from build123d import *
from build123d.topology import SkipClean

# Parameters (mm, degrees)
BOSS_EXTRUDE1_DEPTH = 12
SKETCH2_R           = 0.5
BOSS_EXTRUDE2_DEPTH = 6
SKETCH3_W           = 80
SKETCH3_H           = 60
BOSS_EXTRUDE3_DEPTH = 5


with BuildPart() as part:
    # Sketch1 → Boss-Extrude1 (new body)
    with BuildSketch(Plane(origin=(19, 0, 0), x_dir=(0, 0, -1), z_dir=(1, 0, 0))):
        with BuildLine():
            Line((-17.5, 6.6), (-15.77498019, 6.6))
            ThreePointArc((-15.77498019, 6.6), (0, 17.1), (15.77498019, 6.6))
            Line((15.77498019, 6.6), (17.5, 6.6))
            ThreePointArc((17.5, 6.6), (24.1, 0), (17.5, -6.6))
            Line((17.5, -6.6), (15.77498019, -6.6))
            ThreePointArc((15.77498019, -6.6), (14.603463036, -8.896564918), (13.1, -10.990905331))
            Line((13.1, -10.990905331), (13.1, -12.489995997))
            ThreePointArc((13.1, -12.489995997), (11.807309956, -13.718506901), (10.4, -14.813844876))
            Line((10.4, -14.813844876), (10.4, -16))
            ThreePointArc((10.4, -16), (9.199137803, -18.899137803), (6.3, -20.1))
            Line((6.3, -20.1), (-6.3, -20.1))
            ThreePointArc((-6.3, -20.1), (-9.199137803, -18.899137803), (-10.4, -16))
            Line((-10.4, -16), (-10.4, -14.813844876))
            ThreePointArc((-10.4, -14.813844876), (-11.807309956, -13.718506901), (-13.1, -12.489995997))
            Line((-13.1, -12.489995997), (-13.1, -10.990905331))
            ThreePointArc((-13.1, -10.990905331), (-14.603463036, -8.896564918), (-15.77498019, -6.6))
            Line((-15.77498019, -6.6), (-17.5, -6.6))
            ThreePointArc((-17.5, -6.6), (-24.1, 0), (-17.5, 6.6))
        make_face()
        with BuildLine():
            Line((10.1, -9.838699101), (10.1, -11.22497216))
            ThreePointArc((10.1, -11.22497216), (8.803462488, -12.268212919), (7.4, -13.162446581))
            Line((7.4, -13.162446581), (7.4, -16))
            ThreePointArc((7.4, -16), (7.077817459, -16.777817459), (6.3, -17.1))
            Line((6.3, -17.1), (-6.3, -17.1))
            ThreePointArc((-6.3, -17.1), (-7.077817459, -16.777817459), (-7.4, -16))
            Line((-7.4, -16), (-7.4, -13.162446581))
            ThreePointArc((-7.4, -13.162446581), (-8.803462488, -12.268212919), (-10.1, -11.22497216))
            Line((-10.1, -11.22497216), (-10.1, -9.838699101))
            ThreePointArc((-10.1, -9.838699101), (-12.269489895, -6.947633965), (-13.632681321, -3.6))
            ThreePointArc((-13.632681321, -3.6), (-14.1, 0), (-13.632681321, 3.6))
            ThreePointArc((-13.632681321, 3.6), (0, 14.1), (13.632681321, 3.6))
            ThreePointArc((13.632681321, 3.6), (14.1, 0), (13.632681321, -3.6))
            ThreePointArc((13.632681321, -3.6), (12.269489895, -6.947633965), (10.1, -9.838699101))
        make_face(mode=Mode.SUBTRACT)
    extrude(amount=-BOSS_EXTRUDE1_DEPTH)

    # Sketch2 → Boss-Extrude2 (add)
    # profile 1 of 2: a face of its own
    with SkipClean():  # the faces are left unmerged after this step: merging them gives an invalid solid
        with BuildSketch(Plane.ZY.offset(-7)):
            with BuildLine():
                Line((17.5, 3.5), (13.658696863, 3.5))
                ThreePointArc((13.658696863, 3.5), (14.1, 0), (13.658696863, -3.5))
                Line((13.658696863, -3.5), (17.5, -3.5))
                ThreePointArc((17.5, -3.5), (21, 0), (17.5, 3.5))
            make_face()
            with Locations(Location((17.5, 0, 0), (0, 0, 270))):
                Circle(SKETCH2_R, mode=Mode.SUBTRACT)
        # profile 2 of 2: a face of its own
        with BuildSketch(Plane.ZY.offset(-7)):
            with BuildLine():
                Line((-13.658696863, 3.5), (-17.5, 3.5))
                ThreePointArc((-17.5, 3.5), (-21, 0), (-17.5, -3.5))
                Line((-17.5, -3.5), (-13.658696863, -3.5))
                ThreePointArc((-13.658696863, -3.5), (-14.1, 0), (-13.658696863, 3.5))
            make_face()
            with Locations(Location((-17.5, 0, 0), (0, 0, 270))):
                Circle(SKETCH2_R, mode=Mode.SUBTRACT)
        extrude(amount=BOSS_EXTRUDE2_DEPTH)

    # Sketch3 → Boss-Extrude3 (add)
    with SkipClean():  # the faces are left unmerged after this step: merging them gives an invalid solid
        with BuildSketch(Plane(origin=(19, 0, 0), x_dir=(0, 0, -1), z_dir=(1, 0, 0))):
            Rectangle(SKETCH3_W, SKETCH3_H)
        extrude(amount=BOSS_EXTRUDE3_DEPTH)


solid = part.part
Can you work these out from the model? Positions are in its coordinate system, mm. A direction names the side the tool comes from. Give positions to 0.01 mm unless a question says otherwise; leave off trailing zeros. Loops run counter-clockwise (first coordinate to the right, second up) from the corner with the lowest first, then second, coordinate; pieces in that order, holes last. Notation, with made-up numbers: (41, -3) - (96, -3) arc R19 cw to (96, 34) - close; hole circle Ø1 at (3.25, 76). An arc over 180 degrees is marked (long way). Answer as a JSON object with one key per item and string values.
Q1. Imagine slicing it at B-B on x = 8.5. Write out the boundary of the cut face in (y, z).
Geometry says:
{"outline": "(-20.1, -6.3) arc R4.1 ccw to (-16, -10.4) - (-14.81, -10.4) arc R18.1 ccw to (-12.49, -13.1) - (-10.99, -13.1) arc R17.1 ccw to (-6.6, -15.77) - (-6.6, -17.5) arc R6.6 ccw to (6.6, -17.5) - (6.6, -15.77) arc R17.1 ccw to (6.6, 15.77) - (6.6, 17.5) arc R6.6 ccw to (-6.6, 17.5) - (-6.6, 15.77) arc R17.1 ccw to (-10.99, 13.1) - (-12.49, 13.1) arc R18.1 ccw to (-14.81, 10.4) - (-16, 10.4) arc R4.1 ccw to (-20.1, 6.3) - close; hole (-17.1, -6.3) arc R1.1 ccw to (-16, -7.4) - (-13.16, -7.4) arc R15.1 ccw to (-11.22, -10.1) - (-9.84, -10.1) arc R14.1 ccw (long way) to (-9.84, 10.1) - (-11.22, 10.1) arc R15.1 ccw to (-13.16, 7.4) - (-16, 7.4) arc R1.1 ccw to (-17.1, 6.3) - close"}
Q2. Imagine slicing it at C-C on z = 33. Write out the boundary of the cut face in (x, y), plus the area to 3 significant figures.
Geometry says:
{"outline": "(19, -30) - (24, -30) - (24, 30) - (19, 30) - close", "area": "300 mm²"}
Q3. Will these pins go through, and if not, where does the flat tip stop? P1, Ø3.5, axis at x = 11.5, z = -1, coming from the -Y side; P2, Ø0.7, axis at x = 14.5, y = -10.5, coming from the +Z side; P3, Ø3, axis at x = 4.5, z = 16.5, coming from the -Y side.
Geometry says:
{"P1": "y = -20.1", "P2": "z = 13.76", "P3": "y = -3.5"}
Q4. Imagine slicing it at A-A on x = 4.5. Write out the boundary of the cut face in (y, z), plus the area to 3 significant figures.
Geometry says:
{"outline": "(-3.5, -17.5) arc R3.5 ccw to (3.5, -17.5) - (3.5, -13.66) arc R14.1 cw to (-3.5, -13.66) - close; (-3.5, 13.66) arc R14.1 cw to (3.5, 13.66) - (3.5, 17.5) arc R3.5 ccw to (-3.5, 17.5) - close; hole circle Ø1 at (0, -17.5); hole circle Ø1 at (0, 17.5)", "area": "86.6 mm²"}
Q5. Imagine slicing it at D-D on y = -23.5. Write out the boundary of the cut face in (x, z).
Geometry says:
{"outline": "(19, -40) - (24, -40) - (24, 40) - (19, 40) - close"}
Q6. Which directions (+Z, -Z, +X, -X, +Y, -Y) give clear straight access to the entire face, cutting with the end or side of a thin tool? Please do faces 1 (the flat face through (13, -6.6, 17)), 2 (the flat face through (4, -3.5, 16)), 3 (the flat face through (13, -6.6, -17)), 4 (the flat face through (19, 7, -17)).
Geometry says:
{"face 1": "+Z, -X, -Y", "face 2": "+Z, -Z, -X, -Y", "face 3": "-Z, -X, -Y", "face 4": "-X"}
Q7. If I drill on L1, parallel to Z at x = 5.4, y = 0; L2, parallel to Y at x = 15, z = 0.5; L3, parallel to Z at x = 11.5, y = -3.5, over which ranges is the centre line in solid material (lowest first)?
Geometry says:
{"L1": "-21 to -18, -17 to -14.1, 14.1 to 17, 18 to 21", "L2": "-20.1 to -17.1, 14.09 to 17.09", "L3": "-23.1 to -13.66, 13.66 to 23.1"}
Q8. If we mould it in two halves opening along Z, with no side actions, what happens to faces 5 (the flat face through (13, -15, -7.4)), 6 (the flat face through (13, 6.6, 17)), 7 (the flat face through (21, 0, -40)), 8 (the cylindrical face through (13.084, -12.282, 8.785))? For each: pulls with the +Z half, pulls with the -Z half, needs draft (parallel to the pull), parting line crosses it, or undercut.
Geometry says:
{"face 5": "undercut", "face 6": "needs draft", "face 7": "pulls with the -Z half", "face 8": "undercut"}
